The model under review builds one solid part; all positions refer to its coordinate system, in mm. Face numbers are marked on the shaded views. A direction names the side the tool comes from. Round coordinates to 2 decimals unless told otherwise and drop trailing zeros. Write each loop counter-clockwise with the first axis right and the second up, starting at its lowest first coordinate (ties: lowest second). Pieces come first, ordered by that corner, then holes. Notation, with made-up numbers: M 59.25,59 L 97.25,59 A17 cw 97.25,69 Z; hole C 48.25,-5 d1. An arc over 180 degrees is marked long. One line per item, written item: value. Start each with the question number.
1) Take a section at C-C, the plane z = 7.5. Write out the cut boundary in (x, y).
2) For P1, Ø4, axis at x = 15.5, z = 4.5, coming from the -Y side; P2, Ø5, axis at x = 26.5, z = 6.5, coming from the +Y side; P3, Ø2.5, axis at y = 7, z = 7.5, coming from the -X side, all flat-tipped, find the tip position at first contact; note any pin that passes through.
3) Take a section at A-A, the plane y = 23. Write out the cut boundary in (x, z).
4) Tool access review of the marked faces 4, 5, 6 and 7: name each direction out of +Z, -Z, +X, -X, +Y, -Y from which nothing blocks a thin tool from reaching the whole face with its end or side.
5) Take a section at D-D, the plane x = 11. Write out the cut boundary in (y, z).
6) Take a section at B-B, the plane x = 34. Write out the cut boundary in (y, z).
7) Wall thickness on probe 1 along X at (y, z) = (21.5, 4.25); probe 2 along X at (y, z) = (5.5, 15.5); probe 3 along Y at (x, z) = (3.5, 10.75): over which ranges is each line inside the solid? List them lowest first.
8) Mouldability with a two-part tool opening along Z and no side actions: class the marked faces 1, 2 and 3 as +Z half, -Z half, draft (parallel to the pull), parting line (faces both ways), or undercut.
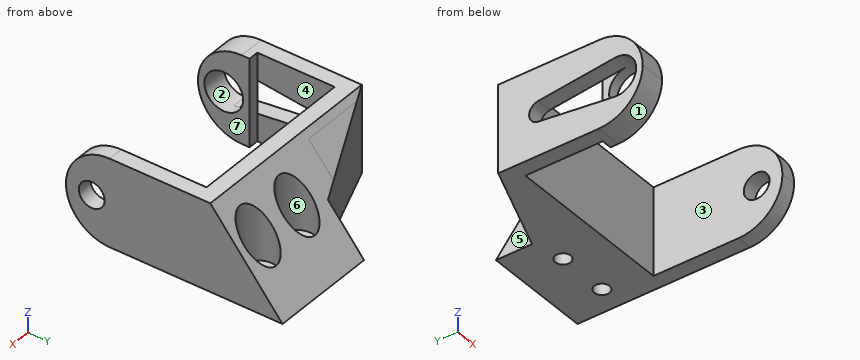
Autodesk Inventor part; units mm, degrees
ref_plane "YZ Plane" through (0, 0, 0) normal (1, 0, 0) x (0, 1, 0)
ref_plane "XZ Plane" through (0, 0, 0) normal (0, 1, 0) x (-1, 0, 0)
ref_plane "XY Plane" through (0, 0, 0) normal (0, 0, 1) x (1, 0, 0)
sketch "Sketch1" plane through (0, 0, 0) normal (0, 0, 1) x (1, 0, 0)
  line L0 (0, 0) -> (5, 0)
  line L1 (5, 0) -> (5, 25)
  line L2 (5, 25) -> (0, 25)
  line L3 (0, 25) -> (0, 0)
  line L4 (36, 25) -> (39, 25)
  line L5 (39, 25) -> (39, 0)
  line L6 (39, 0) -> (36, 0)
  line L7 (36, 0) -> (36, 25)
  line L8 (0, 25) -> (39, 25)
  line L9 (39, 25) -> (39, 42)
  line L10 (39, 42) -> (0, 42)
  line L11 (0, 42) -> (0, 25)
  line L12 (5, 25) -> (3, 25)
  line L13 (3, 25) -> (3, 10)
  line L14 (3, 10) -> (5, 10)
  line L15 (5, 10) -> (5, 25)
  dimension "d0" = 5
  dimension "d1" = 25
  dimension "d2" = 3
  dimension "d3" = 25
  dimension "d4" = 31
  dimension "d6" = 17
  dimension "d48" = 0
  dimension "d54" = 2
  dimension "d55" = 15
extrude "Extrusion1" add sketch "Sketch1" along normal blind 17 contours L3 L2 L13 L14 L1 L0 | L11 L10 L9 L4 L8 L2 | L4 L5 L6 L7
sketch "Sketch2" plane through (39, 0, 0) normal (1, 0, 0) x (0, 0, -1)
  line L0 (-17, 28) -> (-17, 42)
  line L1 (0, 42) -> (-17, 42)
  line L2 (-17, 42) -> (0, 42)
  line L3 (0, 42) -> (-17, 28)
  point P0 (0, 0)
  dimension "d9" = 14
extrude "Extrusion2" cut sketch "Sketch2" against normal up to surface (39 mm away)
sketch "Sketch3" plane through (0, 0, 0) normal (0, 0, -1) x (-1, 0, 0)
  line L0 (0, 42) -> (0, 0)
  line L1 (0, 42) -> (-15, 42)
  line L2 (-15, 42) -> (-15, 29)
  line L3 (-15, 29) -> (0, 29)
  line L4 (0, 29) -> (0, 42)
  point P0 (0, 29)
  dimension "d12" = 15
  dimension "d13" = 13
extrude "Extrusion3" cut sketch "Sketch3" against normal up to surface (17 mm away)
sketch "Sketch4" plane through (0, 0, 17) normal (0, 0, 1) x (1, 0, 0)
  line L0 (39, 0) -> (39, 42)
  line L1 (39, 42) -> (19, 42)
  line L2 (19, 42) -> (19, 25)
  line L3 (19, 25) -> (39, 25)
  line L4 (39, 25) -> (39, 42)
  circle A0 centre (34, 33.5) radius 3.5
  circle A1 centre (24, 33.5) radius 3.5
  point P0 (0, 0)
  dimension "d16" = 20
  dimension "d17" = 17
  dimension "d18" = 7
  dimension "d19" = 7
  dimension "d20" = 8.5
  dimension "d21" = 5
  dimension "d22" = 8.5
  dimension "d23" = 5
extrude "Extrusion4" cut sketch "Sketch4" against normal blind 14 contours A0 | A1
sketch "Sketch5" plane through (0, 0, 3) normal (0, 0, 1) x (1, 0, 0)
  circle A0 centre (34, 33.5) radius 3.5
  circle A1 centre (34, 33.5) radius 1.5
  circle A2 centre (24, 33.5) radius 3.5
  circle A3 centre (24, 33.5) radius 1.5
  point P0 (0, 0)
  point P1 (32.4191, 39.5294)
  point P2 (27.5809, 39.5294)
  point P3 (22.4191, 39.5294)
  point P4 (17.5809, 39.5294)
  dimension "d26" = 3
  dimension "d27" = 3
extrude "Extrusion5" cut sketch "Sketch5" against normal up to surface (3 mm away) contours A1 | A3
sketch "Sketch6" plane through (15, 29, 0) normal (-1, 0, 0) x (0, 0, 1)
  line L0 (0, 0) -> (15.7857, 0)
  line L1 (0, 13) -> (15.7857, 0)
  line L2 (15.7857, 0) -> (0, 0)
  line L3 (0, 0) -> (0, 13)
  line L4 (0, 0) -> (0, 13)
  point P0 (0, -29)
extrude "Extrusion6" add sketch "Sketch6" along normal up to surface (15 mm away)
sketch "Sketch7" plane through (0, 0, 17) normal (0, 0, 1) x (1, 0, 0)
  line L0 (39, 28) -> (0, 28)
  line L1 (0, 28) -> (18, 28)
  line L2 (18, 28) -> (18, 35)
  line L3 (18, 35) -> (0, 28)
  line L4 (18, 35) -> (18, 42)
  line L5 (0, 28) -> (0, 42)
  line L6 (18, 42) -> (0, 42)
  line L7 (0, 42) -> (0, 28)
  point P0 (0, 0)
  dimension "d32" = 18
  dimension "d33" = 7
  dimension "d34" = 7
extrude "Extrusion7" cut sketch "Sketch7" against normal up to surface (17 mm away) contours L5 L6 L4 L3
sketch "Sketch8" plane through (0, 0, 0) normal (-1, 0, 0) x (0, 0, 1)
  circle A0 centre (8.5, 5) radius 3.75
  line L0 (0, 0) -> (17, 0)
  line L1 (17, 28) -> (17, 0)
  dimension "d37" = 7.5
  dimension "d38" = 5
  dimension "d39" = 8.5
extrude "Extrusion8" cut sketch "Sketch8" against normal up to surface (5 mm away)
sketch "Sketch9" plane through (39, 0, 17) normal (1, 0, 0) x (0, 0, -1)
  circle A0 centre (8.5, 5) radius 2.5
  line L0 (17, 0) -> (0, 0)
  line L1 (0, 0) -> (0, 28)
  dimension "d42" = 5
  dimension "d43" = 5
  dimension "d44" = 8.5
extrude "Extrusion9" cut sketch "Sketch9" against normal up to surface (3 mm away)
fillet "Fillet1" radius 8.5 4 edges at (2.5, 0, 17) (37.5, 0, 17) (37.5, 0, 0) (2.5, 0, 0)
sketch "Sketch10" plane through (0, 28, 0) normal (-1, 0, 0) x (0, 0, 1)
  circle A0 centre (8.5, -8) radius 2
  circle A1 centre (8.5, -23) radius 3.75
  line L0 (10.4863, -7.7667) -> (12.2244, -22.5625)
  line L1 (6.5137, -7.7667) -> (4.7756, -22.5625)
  circle A2 centre (8.5, -23) radius 3.75
  circle A3 centre (8.5, -23) radius 3.5
  point P0 (0, -28)
  dimension "d49" = 4
  dimension "d50" = 15
  dimension "d51" = 0
extrude "Extrusion10" cut sketch "Sketch10" against normal blind 3 contours A0 | A0 L0 A1 L1
properties part number "juncao7"
Checked values:
1. outline: M 0,0.06 L 5,0.06 L 5,1.39 L 0,1.39 Z; M 0,21.73 L 3,21.73 L 3,25 L 36,25 L 36,7.29 L 39,7.29 L 39,35.82 L 36.62,35.82 A3.5 cw long 31.38,35.82 L 26.62,35.82 A3.5 cw long 21.38,35.82 L 18,35.82 L 18,35 L 0,28 Z; M 3,8.61 L 5,8.61 L 5,10 L 3,10 Z; M 36,0.06 L 39,0.06 L 39,2.71 L 36,2.71 Z
2. P1: stops at y = 25
2. P2: stops at y = 38.71
2. P3: stops at x = 36
3. outline: M 0,0 L 3,0 L 3,17 L 0,17 Z; M 36,0 L 39,0 L 39,17 L 36,17 Z
4. face 4: +Z, -Z
4. face 5: +Z, -Z, -X, +Y
4. face 6: +Z
4. face 7: +Z, -Z, -Y
5. outline: M 25,0 L 32.28,0 L 32.28,11.81 L 29,15.79 L 28,17 L 25,17 Z
6. outline: M 25,0 L 32,0 L 32,3 L 30,3 L 30,14.57 L 28,17 L 25,17 Z; M 35,0 L 42,0 L 37,6.07 L 37,3 L 35,3 Z
7. probe 1: x = 0 to 3, 36 to 39
7. probe 2: x = 0 to 5, 36 to 39
7. probe 3: y = 0.3 to 2, 8 to 10, 25 to 29.36
8. face 1: -Z half
8. face 2: undercut
8. face 3: draft
